Build history of the part. All positions in model axes, mm. Face numbers are marked on the shaded views. A direction names the side the tool comes from. Give positions to 0.01 mm unless a question says otherwise; leave off trailing zeros. Loops run counter-clockwise (first coordinate to the right, second up) from the corner with the lowest first, then second, coordinate; pieces in that order, holes last. Notation, with made-up numbers: (-17, -8.75) -> (42, -8.75) arc R11 cw to (42, 10.25) -> close; hole circle Ø9 at (-20.5, 39.5). An arc over 180 degrees is marked (long way). Answer as a JSON object with one key per item and string values. Group by question number.
Q1. Band-saw the part on A-A, the plane y = 0. Write the cut outline in (x, z), plus the area to 3 significant figures.
Q2. Tool access for the marked faces 1, 2 and 3: list every direction of +Z, -Z, +X, -X, +Y, -Y with a clear straight run to the whole face (end or side of a thin tool).
Q3. Wall check: probe 1 along Y at (x, z) = (0, 1.3); probe 2 along Y at (x, z) = (28, 0.55); probe 3 along X at (y, z) = (23, 1.45). Give the ranges that are in metal, low to high. Write a range as from..to.
Q4. Two-plate mould, pull along X, no slides. Class the marked faces 4, 5, 6 and 7: pulls with the +X half, pulls with the -X half, needs draft (parallel to the pull), parting line crosses it, or undercut.
Q5. Band-saw the part on D-D, the plane x = -16.5. Write the cut outline in (y, z), plus the area to 3 significant figures.
Q6. Drop flat-ended pins along their axis: pin 1 (2 mm diameter, centred on y = 23, z = 4, fed in from -X); pin 2 (1.5 mm diameter, centred on y = 14.5, z = 1, fed in from -X); pin 3 (4.5 mm diameter, centred on x = 0, y = 0, fed in from -Z); pin 4 (2.5 mm diameter, centred on y = -24.5, z = 2, fed in from -X). Give the stop position or say it passes through.
Q7. Band-saw the part on C-C, the plane y = 20.5. Write the cut outline in (x, z).
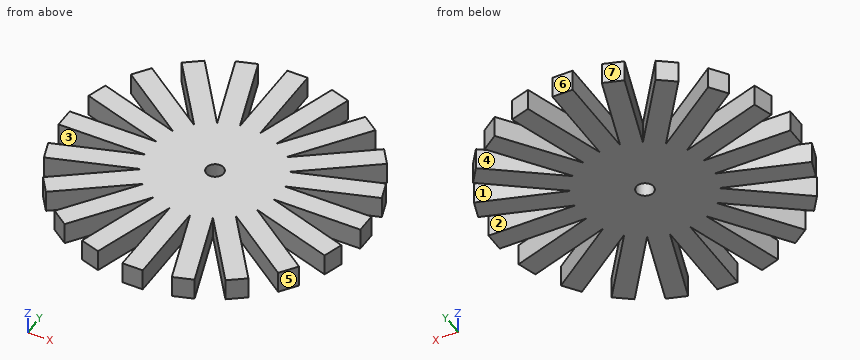
from build123d import *

# Parameters (mm, degrees)
ESQUISSE1_R        = 2
BOSS_EXTRU_1_DEPTH = 5


with BuildPart() as part:
    # Esquisse1 → Boss.-Extru.1 (new body)
    with BuildSketch(Plane.XY):
        Polygon((-14.815325109, -2.346516976), (-34.815325109, -2.346516976), (-34.815325109, 2.346516976), (-14.815325109, 2.346516976), (-33.836455435, 8.526856863), (-32.386228189, 12.990197384), (-13.365097863, 6.809857496), (-29.54543775, 18.565562542), (-26.786941605, 22.362306764), (-10.606601718, 10.606601718), (-22.362306764, 26.786941605), (-18.565562542, 29.54543775), (-6.809857496, 13.365097863), (-12.990197384, 32.386228189), (-8.526856863, 33.836455435), (-2.346516976, 14.815325109), (-2.346516976, 34.815325109), (2.346516976, 34.815325109), (2.346516976, 14.815325109), (8.526856863, 33.836455435), (12.990197384, 32.386228189), (6.809857496, 13.365097863), (18.565562542, 29.54543775), (22.362306764, 26.786941605), (10.606601718, 10.606601718), (26.786941605, 22.362306764), (29.54543775, 18.565562542), (13.365097863, 6.809857496), (32.386228189, 12.990197384), (33.836455435, 8.526856863), (14.815325109, 2.346516976), (34.815325109, 2.346516976), (34.815325109, -2.346516976), (14.815325109, -2.346516976), (33.836455435, -8.526856863), (32.386228189, -12.990197384), (13.365097863, -6.809857496), (29.54543775, -18.565562542), (26.786941605, -22.362306764), (10.606601718, -10.606601718), (22.362306764, -26.786941605), (18.565562542, -29.54543775), (6.809857496, -13.365097863), (12.990197384, -32.386228189), (8.526856863, -33.836455435), (2.346516976, -14.815325109), (2.346516976, -34.815325109), (-2.346516976, -34.815325109), (-2.346516976, -14.815325109), (-8.526856863, -33.836455435), (-12.990197384, -32.386228189), (-6.809857496, -13.365097863), (-18.565562542, -29.54543775), (-22.362306764, -26.786941605), (-10.606601718, -10.606601718), (-26.786941605, -22.362306764), (-29.54543775, -18.565562542), (-13.365097863, -6.809857496), (-32.386228189, -12.990197384), (-33.836455435, -8.526856863), align=None)
        Circle(ESQUISSE1_R, mode=Mode.SUBTRACT)
    extrude(amount=BOSS_EXTRU_1_DEPTH)


solid = part.part
Worked answers:
{
 "1": {"outline": "(-34.82, 0) -> (-2, 0) -> (-2, 5) -> (-34.82, 5) -> close; (2, 0) -> (34.82, 0) -> (34.82, 5) -> (2, 5) -> close", "area": "328 mm2"},
 "2": {"face 1": "+Z, -Z", "face 2": "+Z, -Z, +X", "face 3": "+Z, -Z, -X"},
 "3": {"probe 1": "-34.82..-2, 2..34.82", "probe 2": "-20.69..-17.44, -11.57..-6.63, -2.35..2.35, 6.63..11.57, 17.44..20.69", "probe 3": "-19.61..-13.81, -9.94..-5.01, -2.35..2.35, 5.01..9.94, 13.81..19.61"},
 "4": {"face 4": "undercut", "face 5": "pulls with the +X half", "face 6": "needs draft", "face 7": "pulls with the -X half"},
 "5": {"outline": "(-26.7, 0) -> (-18.72, 0) -> (-18.72, 5) -> (-26.7, 5) -> close; (-14.89, 0) -> (-9.09, 0) -> (-9.09, 5) -> (-14.89, 5) -> close; (-7.83, 0) -> (-2.89, 0) -> (-2.89, 5) -> (-7.83, 5) -> close; (-2.35, 0) -> (2.35, 0) -> (2.35, 5) -> (-2.35, 5) -> close; (2.89, 0) -> (7.83, 0) -> (7.83, 5) -> (2.89, 5) -> close; (9.09, 0) -> (14.89, 0) -> (14.89, 5) -> (9.09, 5) -> close; (18.72, 0) -> (26.7, 0) -> (26.7, 5) -> (18.72, 5) -> close", "area": "211 mm2"},
 "6": {"pin 1": "x = -27.05", "pin 2": "x = -24.98", "pin 3": "z = 0", "pin 4": "x = -21.61"},
 "7": {"outline": "(-28.14, 0) -> (-24.22, 0) -> (-24.22, 5) -> (-28.14, 5) -> close; (-17.79, 0) -> (-11.99, 0) -> (-11.99, 5) -> (-17.79, 5) -> close; (-9.13, 0) -> (-4.19, 0) -> (-4.19, 5) -> (-9.13, 5) -> close; (-2.35, 0) -> (2.35, 0) -> (2.35, 5) -> (-2.35, 5) -> close; (4.19, 0) -> (9.13, 0) -> (9.13, 5) -> (4.19, 5) -> close; (11.99, 0) -> (17.79, 0) -> (17.79, 5) -> (11.99, 5) -> close; (24.22, 0) -> (28.14, 0) -> (28.14, 5) -> (24.22, 5) -> close"}
}
